For this review, take the finished solid that the model builds, in its own axes (mm). A direction names the side the tool comes from. Round coordinates to 2 decimals unless told otherwise and drop trailing zeros. Order: outer loops, then holes, each group sorted by start corner. A loop starts at its lowest first (then second) coordinate and runs counter-clockwise, first axis right, second up. Notation, with made-up numbers: M 49,75.25 L 55,75.25 A15 ccw 55,102.25 Z; hole C -30,44 d8. An arc over 180 degrees is marked long. Answer as a JSON object with one key per item and string values.
from build123d import *
from build123d.topology import SkipClean

# Parameters (mm, degrees)
BOSS_EXTRUDE1_DEPTH      = 19.75
FILLET1_RADIUS           = 9.875
FILLET1_LENGTH           = 48
SKETCH2_R                = 7.55
CUT_EXTRUDE1_DEPTH       = 70.718810231
BOSS_EXTRUDE2_START      = -23
SKETCH3_R                = 6.2
BOSS_EXTRUDE2_DEPTH      = 23
SKETCH4_R                = 4.2
CUT_EXTRUDE2_DEPTH       = 56.624185387
SKETCH5_W                = 7
SKETCH5_H                = 6.5
CUT_EXTRUDE3_DEPTH       = 56.624185387
BOSS_EXTRUDE3_DEPTH      = 4
CUT_EXTRUDE4_START       = -13.5
CUT_EXTRUDE4_OUTLINE_W   = 6.5
CUT_EXTRUDE4_OUTLINE_H   = 7.7
CUT_EXTRUDE4_DEPTH       = 13.5
BOSS_EXTRUDE4_DEPTH      = 5.5
SKETCH9_W                = 6.5
SKETCH9_H                = 7.7
CUT_EXTRUDE5_DEPTH       = 14
BOSS_EXTRUDE5_DEPTH      = 4
BOSS_EXTRUDE6_REACH      = 53.302
SKETCH11_R               = 4.25
CUT_EXTRUDE7_DEPTH       = 55.36094646
CUT_EXTRUDE7_DEPTH_BACK  = 5
SKETCH13_W               = 8.5
SKETCH13_H               = 5.1
CUT_EXTRUDE8_DEPTH       = 2.5
CUT_EXTRUDE6_REACH       = 56.361
SKETCH12_R               = 2.6
BOSS_EXTRUDE7_REACH      = 45.123
BOSS_EXTRUDE7_END_RADIUS = 9.875
SKETCH17_W               = 2.341574484
SKETCH17_H               = 1
CUT_EXTRUDE9_DEPTH       = 70.718810231
BOSS_EXTRUDE8_START      = -1
BOSS_EXTRUDE8_DEPTH      = 0.5
LPATTERN1_COUNT          = 7
LPATTERN1_PITCH          = 7.75
SKETCH19_R               = 4.5
CUT_EXTRUDE10_DEPTH      = 2.5
SKETCH20_W               = 4
SKETCH20_H               = 15.5
BOSS_EXTRUDE9_DEPTH      = 6.45
CUT_EXTRUDE11_REACH      = 44.782
SKETCH22_R               = 4.2
CUT_EXTRUDE12_DEPTH      = 60.71568052


# Read off the part's stored shape, not the designer's step: Cut-Extrude4
with BuildPart() as part:
    # Sketch1 → Boss-Extrude1 (new body)
    with BuildSketch(Plane(origin=(0, 0, 0), x_dir=(1, 0, 0), z_dir=(0, 1, 0))):
        with BuildLine():
            Line((16.074136013, -31.9), (6.75, -31.9))
            Line((6.75, -31.9), (6.75, -38.4))
            Line((6.75, -38.4), (8, -38.4))
            Line((8, -38.4), (8, -42.4))
            Line((8, -42.4), (-8, -42.4))
            Line((-8, -42.4), (-8, -38.4))
            Line((-8, -38.4), (-6.75, -38.4))
            Line((-6.75, -38.4), (-6.75, -31.9))
            Line((-6.75, -31.9), (-16.074136013, -31.9))
            ThreePointArc((-16.074136013, -31.9), (-26.076909961, -33.082331313), (-24, -23.226376819))
            Line((-24, -23.226376819), (-24, 0))
            Line((-24, 0), (24, 0))
            Line((24, 0), (24, -23.226376819))
            ThreePointArc((24, -23.226376819), (26.076909961, -33.082331313), (16.074136013, -31.9))
        make_face()
    extrude(amount=BOSS_EXTRUDE1_DEPTH)

    # Fillet1: full round fillet: the end face becomes a half cylinder, R = half its width
    fillet1_face = Plane((0, 9.875, 0), x_dir=(1, 0, 0), z_dir=(0, 0, -1))  # on the end face: x along it, z out of the body
    fillet1_slab = fillet1_face.offset(-FILLET1_RADIUS / 2) * Box(FILLET1_LENGTH, 2 * FILLET1_RADIUS, FILLET1_RADIUS, mode=Mode.PRIVATE)  # the body's end, R deep
    fillet1_round = Plane((0, 9.875, 9.875), x_dir=(0, 0, -1), z_dir=(1, 0, 0)) * Cylinder(FILLET1_RADIUS, FILLET1_LENGTH, mode=Mode.PRIVATE)  # its axis R under the face
    add(fillet1_slab - fillet1_round, mode=Mode.SUBTRACT)

    # Sketch2 → Cut-Extrude1 (cut, through all)
    with BuildSketch(Plane(origin=(24, 0, 0), x_dir=(0, 0, -1), z_dir=(1, 0, 0))):
        with Locations((-9.875, 9.875)):
            Circle(SKETCH2_R)
    extrude(amount=-CUT_EXTRUDE1_DEPTH, mode=Mode.SUBTRACT)

    # Sketch3 → Boss-Extrude2 (add)
    with SkipClean():  # the faces are left unmerged after this step: merging them gives an invalid solid
        with BuildSketch(Plane(origin=(0, 19.75, 0), x_dir=(1, 0, 0), z_dir=(0, 1, 0)).offset(BOSS_EXTRUDE2_START)):
            with Locations(Location((21.5, -28.9, 0), (0, 0, 66.220005269))):
                Circle(SKETCH3_R)
            with Locations(Location((-21.5, -28.9, 0), (0, 0, 113.779994731))):
                Circle(SKETCH3_R)
        extrude(amount=BOSS_EXTRUDE2_DEPTH)

    # Sketch4 → Cut-Extrude2 (cut, through all)
    with SkipClean():  # the faces are left unmerged after this step: merging them gives an invalid solid
        with BuildSketch(Plane(origin=(0, 19.75, 0), x_dir=(1, 0, 0), z_dir=(0, 1, 0))):
            with Locations(Location((-21.5, -28.9, 0), (0, 0, 270))):
                Circle(SKETCH4_R)
            with Locations(Location((21.5, -28.9, 0), (0, 0, 270))):
                Circle(SKETCH4_R)
        extrude(amount=-CUT_EXTRUDE2_DEPTH, mode=Mode.SUBTRACT)

    # Sketch5 → Cut-Extrude3 (cut, through all)
    with SkipClean():  # the faces are left unmerged after this step: merging them gives an invalid solid
        with BuildSketch(Plane(origin=(0, 19.75, 0), x_dir=(1, 0, 0), z_dir=(0, 1, 0))):
            with Locations((0, -23.15)):
                Rectangle(SKETCH5_W, SKETCH5_H)
            with Locations((0, -35.15)):
                Rectangle(SKETCH5_W, SKETCH5_H)
            with BuildLine():
                Line((17, -19.9), (7, -19.9))
                Line((7, -19.9), (7, -26.4))
                Line((7, -26.4), (8, -26.4))
                Line((8, -26.4), (8, -27.9))
                Line((8, -27.9), (15.381176584, -27.9))
                ThreePointArc((15.381176584, -27.9), (15.945284357, -26.145887779), (17, -24.635026378))
                Line((17, -24.635026378), (17, -19.9))
            make_face()
            with BuildLine():
                Line((-7, -19.9), (-17, -19.9))
                Line((-17, -19.9), (-17, -24.635026378))
                ThreePointArc((-17, -24.635026378), (-15.945284357, -26.145887779), (-15.381176584, -27.9))
                Line((-15.381176584, -27.9), (-8, -27.9))
                Line((-8, -27.9), (-8, -26.4))
                Line((-8, -26.4), (-7, -26.4))
                Line((-7, -26.4), (-7, -19.9))
            make_face()
        extrude(amount=-CUT_EXTRUDE3_DEPTH, mode=Mode.SUBTRACT)

    # Sketch6 → Boss-Extrude3 (add)
    with SkipClean():  # the faces are left unmerged after this step: merging them gives an invalid solid
        with BuildSketch(Plane.XY.offset(42.4)):
            with BuildLine():
                Line((-8, 0), (-8, -1.25))
                ThreePointArc((-8, -1.25), (0, -9.25), (8, -1.25))
                Line((8, -1.25), (8, 0))
                Line((8, 0), (-8, 0))
            make_face()
        extrude(amount=-BOSS_EXTRUDE3_DEPTH)

    # Cut-Extrude4 outline → Cut-Extrude4 (cut)
    with SkipClean():  # the faces are left unmerged after this step: merging them gives an invalid solid
        with BuildSketch(Plane(origin=(6.75, 0, 0), x_dir=(0, 0, -1), z_dir=(1, 0, 0)).offset(CUT_EXTRUDE4_START)):
            with Locations((-35.15, 3.85)):
                Rectangle(CUT_EXTRUDE4_OUTLINE_W, CUT_EXTRUDE4_OUTLINE_H)
        extrude(amount=CUT_EXTRUDE4_DEPTH, mode=Mode.SUBTRACT)
    add(part.part.scale(1), mode=Mode.REPLACE)  # the faces are merged on a copy

    # Sketch8 → Boss-Extrude4 (add)
    with BuildSketch(Plane.XY.offset(31.9)):
        with BuildLine():
            Line((-8, -1.25), (-8, 0))
            Line((-8, 0), (8, 0))
            Line((8, 0), (8, -1.25))
            ThreePointArc((8, -1.25), (0, -9.25), (-8, -1.25))
        make_face()
    extrude(amount=-BOSS_EXTRUDE4_DEPTH)

    # Sketch9 → Cut-Extrude5 (cut)
    with BuildSketch(Plane(origin=(7, 0, 0), x_dir=(0, 0, -1), z_dir=(1, 0, 0))):
        with Locations((-23.15, 3.85)):
            Rectangle(SKETCH9_W, SKETCH9_H)
    extrude(amount=-CUT_EXTRUDE5_DEPTH, mode=Mode.SUBTRACT)

    # Sketch10 → Boss-Extrude5 (add)
    with BuildSketch(Plane.XY.offset(19.9)):
        with BuildLine():
            Line((-8, -1.25), (-8, 0))
            Line((-8, 0), (8, 0))
            Line((8, 0), (8, -1.25))
            ThreePointArc((8, -1.25), (0, -9.25), (-8, -1.25))
        make_face()
    extrude(amount=-BOSS_EXTRUDE5_DEPTH)

    # Boss-Extrude6: up to this face of the body (flat: up to its plane)
    boss_extrude6_end = Plane(part.part.faces().sort_by_distance((0, 13.725, 19.9))[0])
    # Sketch11 → Boss-Extrude6 (add, up to the picked face)
    with BuildSketch(Plane(origin=(0, 0, 38.4), x_dir=(-1, 0, 0), z_dir=(0, 0, -1)), mode=Mode.PRIVATE) as boss_extrude6_sk1:
        with Locations(Location((0, -1.25, 0), (0, 0, 180))):
            Circle(SKETCH11_R)
    boss_extrude6_tool1 = split(extrude(boss_extrude6_sk1.sketch, amount=BOSS_EXTRUDE6_REACH, mode=Mode.PRIVATE), bisect_by=boss_extrude6_end, keep=Keep.BOTH, mode=Mode.PRIVATE)
    add(boss_extrude6_tool1.solids().sort_by(Axis((0, -1.25, 38.4), (0, 0, -1)))[0])

    # Sketch13 → Cut-Extrude7 (cut, two sides: drawn at the far end of the back side and taken through both)
    with BuildSketch(Plane.XZ.offset(-CUT_EXTRUDE7_DEPTH_BACK)):
        with Locations((0, 35.15)):
            Rectangle(SKETCH13_W, SKETCH13_H)
        with Locations((0, 23.15)):
            Rectangle(SKETCH13_W, SKETCH13_H)
    extrude(amount=CUT_EXTRUDE7_DEPTH + CUT_EXTRUDE7_DEPTH_BACK, mode=Mode.SUBTRACT)

    # Sketch15 → Cut-Extrude8 (cut, symmetric)
    with BuildSketch(Plane(origin=(0, 0, 0), x_dir=(0, 0, -1), z_dir=(1, 0, 0))):
        with BuildLine():
            Line((-15.9, 0), (-15.9, 2.050998466))
            ThreePointArc((-15.9, 2.050998466), (-13.05726412, 0.526801239), (-9.875, 0))
            Line((-9.875, 0), (-15.9, 0))
        make_face()
    extrude(amount=CUT_EXTRUDE8_DEPTH, both=True, mode=Mode.SUBTRACT)

    # Cut-Extrude6: up to this face of the body (flat: up to its plane)
    cut_extrude6_end = Plane(part.part.faces().sort_by_distance((0, -3.978206263, 15.9))[0])
    # Sketch12 → Cut-Extrude6 (cut, up to the picked face)
    with BuildSketch(Plane.XY.offset(42.4), mode=Mode.PRIVATE) as cut_extrude6_sk1:
        with Locations((0, -1.25)):
            Circle(SKETCH12_R)
    cut_extrude6_tool1 = split(extrude(cut_extrude6_sk1.sketch, amount=-CUT_EXTRUDE6_REACH, mode=Mode.PRIVATE), bisect_by=cut_extrude6_end, keep=Keep.BOTH, mode=Mode.PRIVATE)
    add(cut_extrude6_tool1.solids().sort_by(Axis((0, -1.25, 42.4), (0, 0, -1)))[0], mode=Mode.SUBTRACT)

    # Boss-Extrude7: up to this cylinder (the profile starts outside it)
    boss_extrude7_end = Plane(origin=(2.389901, 9.875, 9.875), z_dir=(1, 0, 0)) * Cylinder(BOSS_EXTRUDE7_END_RADIUS, 110.996, mode=Mode.PRIVATE)
    # Sketch16 → Boss-Extrude7 (add, up to the surface)
    with BuildSketch(Plane(origin=(0, 0, 15.9), x_dir=(-1, 0, 0), z_dir=(0, 0, -1)), mode=Mode.PRIVATE) as boss_extrude7_sk1:
        with BuildLine():
            Line((-2.279802623, 0), (-2.5, 0))
            Line((-2.5, 0), (-2.5, 1.800187721))
            Line((-2.5, 1.800187721), (2.5, 1.800187721))
            Line((2.5, 1.800187721), (2.5, 0))
            Line((2.5, 0), (2.279802623, 0))
            ThreePointArc((2.279802623, 0), (0, 1.35), (-2.279802623, 0))
        make_face()
    boss_extrude7_tool1 = extrude(boss_extrude7_sk1.sketch, amount=BOSS_EXTRUDE7_REACH, mode=Mode.PRIVATE) - boss_extrude7_end
    add(boss_extrude7_tool1.solids().sort_by_distance((2.389901, 0.053142, 15.9))[0])

    # Sketch17 → Cut-Extrude9 (cut, through all)
    with BuildSketch(Plane.ZY.offset(24)):
        with Locations((1.170787242, 9.875)):
            Rectangle(SKETCH17_W, SKETCH17_H)
    extrude(amount=-CUT_EXTRUDE9_DEPTH, mode=Mode.SUBTRACT)

    # Sketch18 → Boss-Extrude8 (add)
    with BuildSketch(Plane.ZY.offset(24).offset(BOSS_EXTRUDE8_START)):
        with BuildLine():
            Line((0.012666351, 10.375), (2.341574484, 10.375))
            ThreePointArc((2.341574484, 10.375), (2.325, 9.875), (2.341574484, 9.375))
            Line((2.341574484, 9.375), (0.012666351, 9.375))
            ThreePointArc((0.012666351, 9.375), (0, 9.875), (0.012666351, 10.375))
        make_face()
    boss_extrude8 = extrude(amount=BOSS_EXTRUDE8_DEPTH)

    # LPattern1: Boss-Extrude8 ×7
    with Locations(*[(i * LPATTERN1_PITCH, 0, 0) for i in range(1, LPATTERN1_COUNT)]):
        add(boss_extrude8)

    # Sketch19 → Cut-Extrude10 (cut)
    with BuildSketch(Plane.XY.offset(42.4)):
        with Locations((0, -1.25)):
            Circle(SKETCH19_R)
    extrude(amount=-CUT_EXTRUDE10_DEPTH, mode=Mode.SUBTRACT)

    # Sketch20 → Boss-Extrude9 (add)
    with BuildSketch(Plane.ZY.offset(24)):
        with Locations((24.65, 12)):
            Rectangle(SKETCH20_W, SKETCH20_H)
    extrude(amount=BOSS_EXTRUDE9_DEPTH)

    # Sketch21 → Cut-Extrude11 (cut, up to next)
    with BuildSketch(Plane(origin=(0, 0, 22.65), x_dir=(-1, 0, 0), z_dir=(0, 0, -1)), mode=Mode.PRIVATE) as cut_extrude11_sk1:
        Polygon((27.4983, 19.75), (30.45, 19.75), (30.45, 15.9032), align=None)
    cut_extrude11_tool1 = extrude(cut_extrude11_sk1.sketch, amount=-CUT_EXTRUDE11_REACH, mode=Mode.PRIVATE) & part.part
    add(cut_extrude11_tool1.solids().sort_by_distance((-29.4661, 18.467733, 22.65))[0], mode=Mode.SUBTRACT)

    # Sketch22 → Cut-Extrude12 (cut, through all)
    with BuildSketch(Plane(origin=(0, 19.75, 0), x_dir=(1, 0, 0), z_dir=(0, 1, 0))):
        with Locations(Location((-21.5, -28.9, 0), (0, 0, 270))):
            Circle(SKETCH22_R)
    extrude(amount=-CUT_EXTRUDE12_DEPTH, mode=Mode.SUBTRACT)


solid = part.part
1) Insertion check: P1, Ø7, axis at x = -0.5, y = 0.5, coming from the -Z side; P2, Ø2, axis at y = 12.5, z = 35.5, coming from the -X side; P3, Ø1, axis at x = 5.5, y = 14, coming from the -Z side. Each pin has a flat end and moves straight along its axis. Give the tip position at first contact, or say it passes through.
Geometry check:
{"P1": "stops at z = 1.94", "P2": "stops at x = -24.16", "P3": "stops at z = 0.69"}
2) Machinability: for faces 1 (the flat face through (19, 9.375, 1)), 2 (the flat face through (-18, -3.25, 26)), 3 (the cylindrical face through (-0.59, 3.21, 41.17)), which of the approach directions +Z, -Z, +X, -X, +Y, -Y give a long, thin tool a straight path to every point of the face, cutting with its end or side? Answer none if there is none.
Geometry check:
{"face 1": "-Z", "face 2": "+Z, -Z, -X, -Y", "face 3": "+Z"}
3) Add section B-B on z = 3. State the section outline as (x, y) points, and give its area (3 significant figures).
Geometry check:
{"outline": "M -24,2.79 L 24,2.79 L 24,6.75 L -24,6.75 Z; M -24,13 L 24,13 L 24,16.96 L -24,16.96 Z", "area": "381 mm²"}
4) Mouldability with a two-part tool opening along Z and no side actions: class faces 4 (the flat face through (2, 1, 37.7)), 5 (the flat face through (-12, 10.375, 1)), 6 (the flat face through (12, 10, 27.9)), 7 (the flat face through (0, 9, 42.4)) as +Z half, -Z half, draft (parallel to the pull), parting line (faces both ways), or undercut.
Geometry check:
{"face 4": "undercut", "face 5": "draft", "face 6": "undercut", "face 7": "+Z half"}
5) For L1, parallel to X at y = 4.25, z = 28.9; L2, parallel to Y at x = 0, z = 31; L3, parallel to X at y = 0.25, z = 26.5, list the stretches that pass through material, from the lowest coordinate up.
Geometry check:
{"L1": "x = -27.7 to -25.7, -17.3 to 17.3, 25.7 to 27.7", "L2": "y = -9.25 to -3.85, 1.35 to 19.75", "L3": "x = -27.22 to -24.95, -18.05 to -15.78, -8 to -2.12, 2.12 to 8, 15.78 to 18.05, 24.95 to 27.22"}
6) Add section C-C on x = 21.5. State the section outline as (y, z) points (3 decimals), and give its area (3 significant figures).
Geometry check:
{"outline": "M -3.25,22.7 L 0,22.7 L 0,9.875 A9.875 ccw 9.375,0.013 L 9.375,2.342 A7.55 cw long 10.375,2.342 L 10.375,0.013 A9.875 ccw 19.75,9.875 L 19.75,24.7 L -3.25,24.7 Z; M -3.25,33.1 L 19.75,33.1 L 19.75,35.1 L -3.25,35.1 Z", "area": "317 mm²"}
7) Add section A-A on x = 10. State the section outline as (y, z) points (3 decimals), and give its area (3 significant figures).
Geometry check:
{"outline": "M 0,9.875 A9.875 ccw 9.375,0.013 L 9.375,2.342 A7.55 cw long 10.375,2.342 L 10.375,0.013 A9.875 ccw 19.75,9.875 L 19.75,19.9 L 0,19.9 Z; M 0,27.9 L 19.75,27.9 L 19.75,31.9 L 0,31.9 Z", "area": "249 mm²"}
8) Add section D-D on z = 9. State the section outline as (x, y) points.
Geometry check:
{"outline": "M -24,0.04 L 24,0.04 L 24,2.38 L -24,2.38 Z; M -24,17.37 L 24,17.37 L 24,19.71 L -24,19.71 Z"}
